```python
from build123d import *

# Parameters (mm, degrees)
F1_DEPTH = 161.925
F2_R     = 2.286
F3_DEPTH = 25.4
F4_R     = 2.5
F5_DEPTH = 25.4


with BuildPart() as f1:
    # F0 (on Top) → F1 (new body, symmetric)
    with BuildSketch(Plane.XY):
        with BuildLine():
            Line((4.318, 2.3876), (-4.318, 2.3876))
            ThreePointArc((-4.318, 2.3876), (-5.9344461018, 1.7180461018), (-6.604, 0.1016))
            Line((-6.604, 0.1016), (-6.604, -0.1016))
            ThreePointArc((-6.604, -0.1016), (-5.9344461018, -1.7180461018), (-4.318, -2.3876))
            Line((-4.318, -2.3876), (4.318, -2.3876))
            ThreePointArc((4.318, -2.3876), (5.9344461018, -1.7180461018), (6.604, -0.1016))
            Line((6.604, -0.1016), (6.604, 0.1016))
            ThreePointArc((6.604, 0.1016), (5.9344461018, 1.7180461018), (4.318, 2.3876))
        make_face()
    extrude(amount=F1_DEPTH, both=True)

    # F2 (on face) → F3 (cut)
    with BuildSketch(Plane.XZ.offset(2.3876)):
        with Locations((0, 156.21)):
            Circle(F2_R)
        with Locations((0, 127.635)):
            Circle(F2_R)
    extrude(amount=-F3_DEPTH, mode=Mode.SUBTRACT)

    # F4 (on face) → F5 (cut)
    with BuildSketch(Plane.XZ.offset(2.3876)):
        with Locations((0, -146.05)):
            Circle(F4_R)
    extrude(amount=-F5_DEPTH, mode=Mode.SUBTRACT)


solid = f1.part
```
Build history of the part. All positions in model axes, mm. Give positions to 0.01 mm unless a question says otherwise; leave off trailing zeros. Order: outer loops, then holes, each group sorted by start corner. A loop starts at its lowest first (then second) coordinate and runs counter-clockwise, first axis right, second up. Notation, with made-up numbers: M -36,37 L 0,37 A14 cw 0,55 Z; hole C 83.25,-18 d7. An arc over 180 degrees is marked long. Write item = value, one per line. Start each with the question number.
(1) Slice it at C-C on z = 82. Write the cut outline in (x, y).
(2) Slice it at A-A on x = 0. Write the cut outline in (y, z) (3 decimals).
(3) Pin check, flat tips, straight feed: pin 1 Ø3.5 at (x, z) = (0, 127.635) entering from -Y; pin 2 Ø5.5 at (x, z) = (0, 156.21) entering from +Y. Stop position of each tip, or through.
(4) Slice it at B-B on y = 0.85. Write the cut outline in (x, z) (3 decimals).
(5) Two-plate mould, pull along X, no slides. Class faces 1 (the cylindrical face through (1.34, -0.03, -143.94)), 2 (the flat face through (0, 2.388, 2)): released by +X, released by -X, zero draft, split by the parting line, or undercut.
(6) Probe L1, parallel to Z at x = 0, y = -0.65 (3 decimals); L2, parallel to X at y = -0.3, z = 156.21; L3, parallel to Z at x = -0.75, y = -0.7 (3 decimals). List the from-to ranges inside material, lowest first. Write a range as [from, to].
Responses:
q1.outline = M -6.6,-0.1 A2.29 ccw -4.32,-2.39 L 4.32,-2.39 A2.29 ccw 6.6,-0.1 L 6.6,0.1 A2.29 ccw 4.32,2.39 L -4.32,2.39 A2.29 ccw -6.6,0.1 Z
q2.outline = M -2.388,-161.925 L 2.388,-161.925 L 2.388,-148.55 L -2.388,-148.55 Z; M -2.388,-143.55 L 2.388,-143.55 L 2.388,125.349 L -2.388,125.349 Z; M -2.388,129.921 L 2.388,129.921 L 2.388,153.924 L -2.388,153.924 Z; M -2.388,158.496 L 2.388,158.496 L 2.388,161.925 L -2.388,161.925 Z
q3.pin_1 = through
q3.pin_2 = 2.39
q4.outline = M -6.478,-161.925 L 6.478,-161.925 L 6.478,161.925 L -6.478,161.925 Z; hole C 0,-146.05 d5; hole C 0,127.635 d4.572; hole C 0,156.21 d4.572
q5.face_1 = undercut
q5.face_2 = zero draft
q6.L1 = [-161.925, -148.55], [-143.55, 125.349], [129.921, 153.924], [158.496, 161.925]
q6.L2 = [-6.6, -2.29], [2.29, 6.6]
q6.L3 = [-161.925, -148.435], [-143.665, 125.476], [129.794, 154.051], [158.369, 161.925]
